Geometry check sheet. Reference: the model listing, model coordinates, mm. Give positions to 0.01 mm unless a question says otherwise; leave off trailing zeros. Write each loop counter-clockwise with the first axis right and the second up, starting at its lowest first coordinate (ties: lowest second). Pieces come first, ordered by that corner, then holes. Notation, with made-up numbers: M 1.5,62 L 58.5,62 A31 cw 58.5,96 Z; hole C 59,62.5 d7. An arc over 180 degrees is marked long. One line per item, written item: value. Start each with the question number.
1. Gauge pin test, flat ends, axial feed: pin 1 (3 mm diameter, centred on x = 178.71, z = -121.8, fed in from +Y); pin 2 (1 mm diameter, centred on y = 0.5, z = -102.5, fed in from +X); pin 3 (3 mm diameter, centred on x = 2.5, z = -121.8, fed in from -Y); pin 4 (0.6 mm diameter, centred on x = 182, y = 1, fed in from -Z). Record the tip position at first contact, or that the pin passes through.
2. Cross-section at B-B on x = 150. Record the cut outline in (y, z), then the cut area to 3 significant figures.
3. Scan lines: line 1 (X direction, y = 1.7, z = -2.5) (3 decimals); line 2 (X direction, y = 1.55, z = -121.8); line 3 (Z direction, x = 148, y = 1.75). Record each from-to range of solid material in increasing order.
4. Cross-section at C-C on z = -19.65. Record the cut outline in (x, y), then the cut area to 3 significant figures.
5. Cross-section at D-D on z = -49. Record the cut outline in (x, y).
6. Cross-section at A-A on z = -104.65. Record the cut outline in (x, y), then the cut area to 3 significant figures.
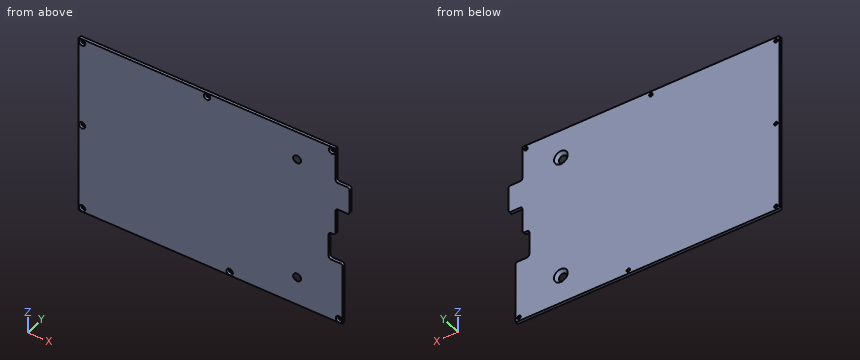
from build123d import *

# Parameters (mm, degrees)
PLATE_FRAME_DEPTH                              = 2
CSK_FOR_M2_FLAT_HEAD_MACHINE_SCREW2_AT_2_COUNT = 2
CSK_FOR_M2_FLAT_HEAD_MACHINE_SCREW2_AT_2_PITCH = 75
CSK_FOR_M2_FLAT_HEAD_MACHINE_SCREW2_AT_3_COUNT = 2
CSK_FOR_M2_FLAT_HEAD_MACHINE_SCREW2_AT_3_PITCH = 176.2125
CSK_FOR_M2_FLAT_HEAD_MACHINE_SCREW2_AT_4_COUNT = 2
CSK_FOR_M2_FLAT_HEAD_MACHINE_SCREW2_AT_4_PITCH = 186.034856025
CSK_FOR_M2_FLAT_HEAD_MACHINE_SCREW2_AT_5_COUNT = 2
CSK_FOR_M2_FLAT_HEAD_MACHINE_SCREW2_AT_5_PITCH = 212.798813804
CSK_FOR_M2_FLAT_HEAD_MACHINE_SCREW2_AT_6_COUNT = 2
CSK_FOR_M2_FLAT_HEAD_MACHINE_SCREW2_AT_6_PITCH = 149.734690891
CSK_FOR_M2_FLAT_HEAD_MACHINE_SCREW2_AT_7_COUNT = 2
CSK_FOR_M2_FLAT_HEAD_MACHINE_SCREW2_AT_7_PITCH = 119.395022535
CSK_FOR_M4_FLAT_HEAD_MACHINE_SCREW1_AT_2_COUNT = 2
CSK_FOR_M4_FLAT_HEAD_MACHINE_SCREW1_AT_2_PITCH = 85
FILLET3_R                                      = 1.5
FILLET4_R                                      = 0.5


with BuildPart() as part:
    # Sketch1 → Plate Frame (new body)
    with BuildSketch(Plane(origin=(0, 0, 0), x_dir=(1, 0, 0), z_dir=(0, 1, 0))):
        Polygon((0, 0), (0, 124.3), (181.2125, 124.3), (181.2125, 81.2), (171.6875, 81.2), (171.6875, 62.15), (176.45, 62.15), (176.45, 43.1), (185.975, 43.1), (185.975, 24.05), (176.45, 24.05), (176.45, 0), align=None)
    extrude(amount=PLATE_FRAME_DEPTH)

    # Sketch23 → CSK for M2 Flat Head Machine Screw2 (revolve, cut)
    with BuildSketch(Plane(origin=(178.7125, 0, -121.8), x_dir=(0, 0, -1), z_dir=(1, 0, 0))):
        Polygon((0, 0), (0, 2), (1.2, 2), (1.2, 1), (2.2, 0), align=None)
    csk_for_m2_flat_head_machine_screw2 = revolve(axis=Axis((178.7125, -6.35, -121.8), (0, 1, 0)), mode=Mode.SUBTRACT)

    # CSK for M2 Flat Head Machine Screw2 at 2: CSK for M2 Flat Head Machine Screw2 ×2
    with Locations(*[(-i * CSK_FOR_M2_FLAT_HEAD_MACHINE_SCREW2_AT_2_PITCH, 0, 0) for i in range(1, CSK_FOR_M2_FLAT_HEAD_MACHINE_SCREW2_AT_2_COUNT)]):
        add(csk_for_m2_flat_head_machine_screw2, mode=Mode.SUBTRACT)

    # CSK for M2 Flat Head Machine Screw2 at 3: CSK for M2 Flat Head Machine Screw2 ×2
    with Locations(*[(-i * CSK_FOR_M2_FLAT_HEAD_MACHINE_SCREW2_AT_3_PITCH, 0, 0) for i in range(1, CSK_FOR_M2_FLAT_HEAD_MACHINE_SCREW2_AT_3_COUNT)]):
        add(csk_for_m2_flat_head_machine_screw2, mode=Mode.SUBTRACT)

    # CSK for M2 Flat Head Machine Screw2 at 4: CSK for M2 Flat Head Machine Screw2 ×2
    with Locations(*[Vector(-0.9472015286011822, 0, 0.3206388376594201) * (i * CSK_FOR_M2_FLAT_HEAD_MACHINE_SCREW2_AT_4_PITCH) for i in range(1, CSK_FOR_M2_FLAT_HEAD_MACHINE_SCREW2_AT_4_COUNT)]):
        add(csk_for_m2_flat_head_machine_screw2, mode=Mode.SUBTRACT)

    # CSK for M2 Flat Head Machine Screw2 at 5: CSK for M2 Flat Head Machine Screw2 ×2
    with Locations(*[Vector(-0.828070875256726, 0, 0.5606234257962827) * (i * CSK_FOR_M2_FLAT_HEAD_MACHINE_SCREW2_AT_5_PITCH) for i in range(1, CSK_FOR_M2_FLAT_HEAD_MACHINE_SCREW2_AT_5_COUNT)]):
        add(csk_for_m2_flat_head_machine_screw2, mode=Mode.SUBTRACT)

    # CSK for M2 Flat Head Machine Screw2 at 6: CSK for M2 Flat Head Machine Screw2 ×2
    with Locations(*[Vector(-0.6043188753487793, 0, 0.7967425537130464) * (i * CSK_FOR_M2_FLAT_HEAD_MACHINE_SCREW2_AT_6_PITCH) for i in range(1, CSK_FOR_M2_FLAT_HEAD_MACHINE_SCREW2_AT_6_COUNT)]):
        add(csk_for_m2_flat_head_machine_screw2, mode=Mode.SUBTRACT)

    # CSK for M2 Flat Head Machine Screw2 at 7: CSK for M2 Flat Head Machine Screw2 ×2
    with Locations(*[Vector(-0.039888597521597645, 0, 0.9992041331918919) * (i * CSK_FOR_M2_FLAT_HEAD_MACHINE_SCREW2_AT_7_PITCH) for i in range(1, CSK_FOR_M2_FLAT_HEAD_MACHINE_SCREW2_AT_7_COUNT)]):
        add(csk_for_m2_flat_head_machine_screw2, mode=Mode.SUBTRACT)

    # Sketch26 → CSK for M4 Flat Head Machine Screw1 (revolve, cut)
    with BuildSketch(Plane(origin=(150, 2, -104.65), x_dir=(0, 0, 1), z_dir=(1, 0, 0))):
        Polygon((0, 0), (0, 2), (2.25, 2), (2.25, 2.45), (4.7, 0), align=None)
    csk_for_m4_flat_head_machine_screw1 = revolve(axis=Axis((150, 8.35, -104.65), (0, -1, 0)), mode=Mode.SUBTRACT)

    # CSK for M4 Flat Head Machine Screw1 at 2: CSK for M4 Flat Head Machine Screw1 ×2
    with Locations(*[(0, 0, i * CSK_FOR_M4_FLAT_HEAD_MACHINE_SCREW1_AT_2_PITCH) for i in range(1, CSK_FOR_M4_FLAT_HEAD_MACHINE_SCREW1_AT_2_COUNT)]):
        add(csk_for_m4_flat_head_machine_screw1, mode=Mode.SUBTRACT)

    # Fillet3
    fillet3_edges = [part.edges().sort_by_distance(p)[0] for p in [
        (181.2125, 1, -81.2),
        (171.6875, 1, -81.2),
        (171.6875, 1, -62.15),
        (176.45, 1, -62.15),
        (176.45, 1, -43.1),
        (185.975, 1, -43.1),
        (185.975, 1, -24.05),
        (176.45, 1, -24.05),
    ]]
    fillet(fillet3_edges, radius=FILLET3_R)

    # Fillet4
    fillet4_edges = [part.edges().sort_by_distance(p)[0] for p in [
        (0, 1, 0),
        (0, 1, -124.3),
        (181.2125, 1, -124.3),
        (176.45, 1, 0),
    ]]
    fillet(fillet4_edges, radius=FILLET4_R)


solid = part.part
Report:
1. pin 1: stops at y = 2
1. pin 2: stops at x = 181.21
1. pin 3: stops at y = 0.7
1. pin 4: stops at z = -43.1
2. outline: M 0,-124.3 L 2,-124.3 L 2,-109.35 L 0,-107.35 Z; M 0,-101.95 L 2,-99.95 L 2,-24.35 L 0,-22.35 Z; M 0,-16.95 L 2,-14.95 L 2,0 L 0,0 Z
2. area: 219 mm^2
3. line 1: x = 0 to 1.3, 3.7 to 87.025, 89.425 to 172.75, 175.15 to 176.45
3. line 2: x = 0 to 1.3, 3.7 to 102.51, 104.91 to 177.51, 179.91 to 181.21
3. line 3: z = -124.3 to -108.63, -100.67 to -23.63, -15.67 to 0
4. outline: M 0,0 L 147.3,0 L 145.3,2 L 0,2 Z; M 152.7,0 L 176.45,0 L 176.45,2 L 154.7,2 Z
4. area: 338 mm^2
5. outline: M 0,0 L 176.45,0 L 176.45,2 L 0,2 Z
6. outline: M 0,0 L 147.3,0 L 145.3,2 L 0,2 Z; M 152.7,0 L 181.21,0 L 181.21,2 L 154.7,2 Z
6. area: 348 mm^2
